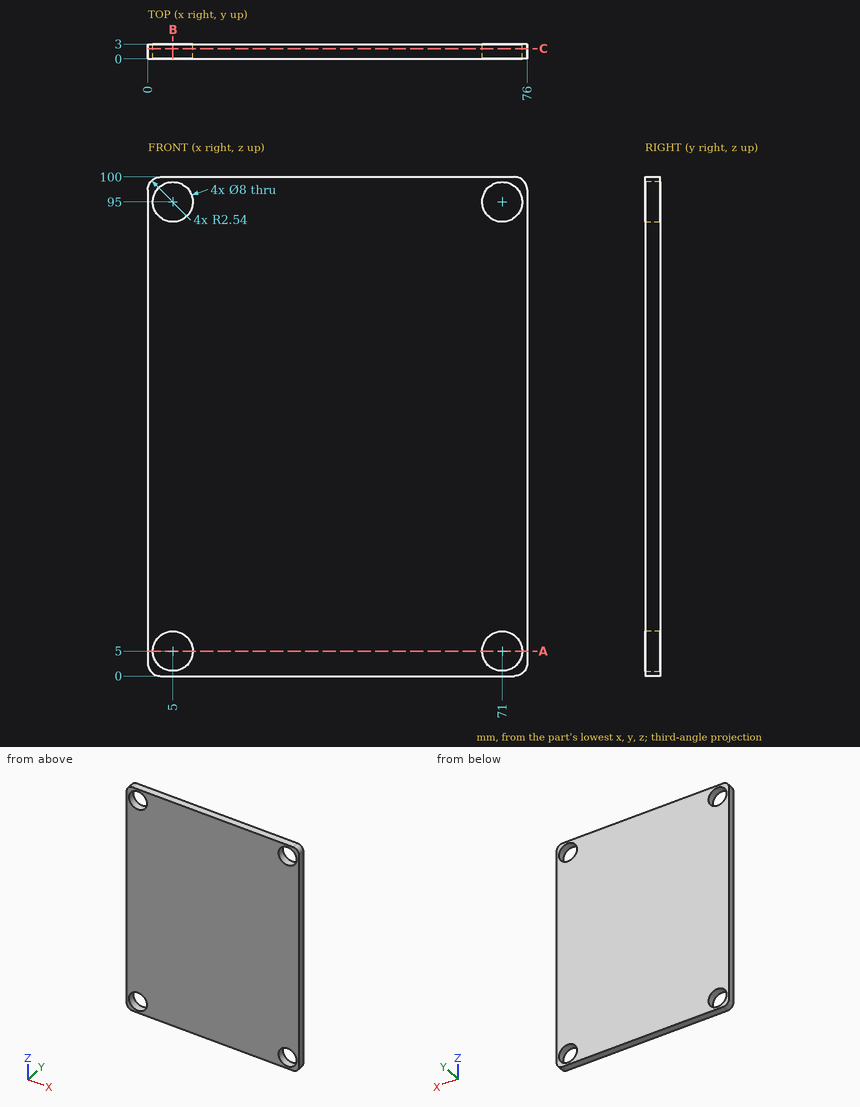
The figure shows three views and two pictorial views of one solid part (mm, origin at its lowest corner). Answer the questions. Give positions to 0.01 mm unless a question says otherwise; leave off trailing zeros. Write each loop counter-clockwise with the first axis right and the second up, starting at its lowest first coordinate (ties: lowest second). Pieces come first, ordered by that corner, then holes. Notation, with made-up numbers: M 7,45.5 L 12,45.5 A13 cw 12,52.5 Z; hole C 35.5,51.5 d5. An arc over 180 degrees is marked long. One line per item, written item: value. Start each with the question number.
(1) Find section B-B (x = 5). Determine the outline of the cut face in (y, z), plus the area to 3 significant figures.
(2) Find section A-A (z = 5). Determine the outline of the cut face in (x, y).
(3) Find the intervals of material crossed by line 1 (X direction, y = 1.1, z = 95); line 2 (Z direction, x = 6, y = 2.05); line 3 (Z direction, x = 72.5, y = 1.95), in increasing order.
(4) Find section C-C (y = 2.05). Determine the outline of the cut face in (x, z).
Results below:
1. outline: M 0,0 L 3,0 L 3,1 L 0,1 Z; M 0,9 L 3,9 L 3,91 L 0,91 Z; M 0,99 L 3,99 L 3,100 L 0,100 Z
1. area: 252 mm^2
2. outline: M 0,0 L 1,0 L 1,3 L 0,3 Z; M 9,0 L 67,0 L 67,3 L 9,3 Z; M 75,0 L 76,0 L 76,3 L 75,3 Z
3. line 1: x = 0 to 1, 9 to 67, 75 to 76
3. line 2: z = 0 to 1.13, 8.87 to 91.13, 98.87 to 100
3. line 3: z = 0 to 1.29, 8.71 to 91.29, 98.71 to 100
4. outline: M 0,2.54 A2.54 ccw 2.54,0 L 73.46,0 A2.54 ccw 76,2.54 L 76,97.46 A2.54 ccw 73.46,100 L 2.54,100 A2.54 ccw 0,97.46 Z; hole C 5,5 d8; hole C 5,95 d8; hole C 71,5 d8; hole C 71,95 d8
